Part model, mm, in its own coordinate system. Face numbers are marked on the shaded views. A direction names the side the tool comes from. Give positions to 0.01 mm unless a question says otherwise; leave off trailing zeros. Order: outer loops, then holes, each group sorted by start corner. A loop starts at its lowest first (then second) coordinate and runs counter-clockwise, first axis right, second up. Notation, with made-up numbers: (48.5, -4) - (75.5, -4) arc R36 cw to (75.5, 34) - close; hole circle Ø5 at (-17.5, 19.25). An arc over 180 degrees is marked (long way). Use one line per item in the form item = value. Start each with the question number.
1. Pull direction X, two halves, no side cores. Call the marked faces 3, 4, 5 and 6: +X half, -X half, draft (parallel to the pull), parting line (faces both ways), or undercut.
2. Band-saw the part on B-B, the plane z = 0. List the corners of the cut face in (x, y).
3. Drill centre lines: line 1 (X direction, y = 21.25, z = 19.05); line 2 (Z direction, x = -10.5, y = 0.25); line 3 (X direction, y = 20.8, z = -38.1). Where is each one in solid material? Low to high.
4. Pin check, flat tips, straight feed: P1, Ø2.5, axis at y = 2.5, z = 33, coming from the +X side; P2, Ø4, axis at y = 2.5, z = 31, coming from the -X side; P3, Ø8, axis at x = 4.5, z = 36, coming from the +Y side; P4, Ø12, axis at x = 18.5, y = 17, coming from the -Z side. Stop position of each tip, or through.
5. Band-saw the part on D-D, the plane z = 30.5. List the corners of the cut face in (x, y) (3 decimals).
6. Tool access for the marked faces 1 and 2: list every direction of +Z, -Z, +X, -X, +Y, -Y with a clear straight run to the whole face (end or side of a thin tool).
7. Band-saw the part on C-C, the plane y = 10.75. State how many separate pieces and enclosed holes the cut face has, plus the area to 3 significant figures.
8. Band-saw the part on A-A, the plane x = 14.5. List the corners of the cut face in (y, z), plus the area to 3 significant figures.
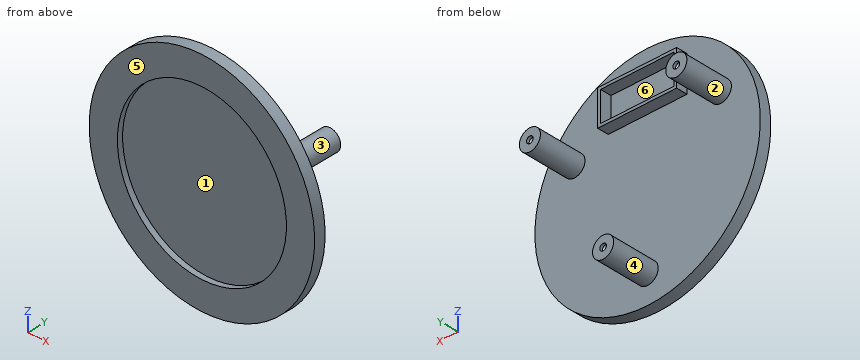
from build123d import *

# Parameters (mm, degrees)
SKETCH3_R                 = 4.7625
BOSS_EXTRUDE1_DEPTH       = 21.59
M4X0_7_TAPPED_HOLE1_D     = 3
M4X0_7_TAPPED_HOLE1_DEPTH = 1.27
M4X0_7_TAPPED_HOLE1_TIP   = 0.901290929
SKETCH12_W                = 35.54
SKETCH12_H                = 16.04
SKETCH12_W_2              = 33
SKETCH12_H_2              = 13.5
BOSS_EXTRUDE2_DEPTH       = 5.08


with BuildPart() as part:
    # Sketch1 → Revolve1 (revolve)
    with BuildSketch(Plane.XY, mode=Mode.PRIVATE) as revolve1_sk:
        Polygon((-38.1, -2.54), (0, -2.54), (0, 0), (-50.8, 0), (-50.8, -5.08), (-38.1, -5.08), align=None)
    revolve(revolve1_sk.sketch.rotate(Axis((0, 4.567685351, 0), (0, -1, 0)), 270), axis=Axis((0, 4.567685351, 0), (0, -1, 0)))

    # Sketch3 → Boss-Extrude1 (add)
    with BuildSketch(Plane(origin=(0, 0, 0), x_dir=(1, 0, 0), z_dir=(0, 1, 0))):
        with Locations(Location((0, 38.1, 0), (0, 0, 270))):
            Circle(SKETCH3_R)
        with Locations(Location((-32.995567884, -19.05, 0), (0, 0, 270))):
            Circle(SKETCH3_R)
        with Locations(Location((32.995567884, -19.05, 0), (0, 0, 270))):
            Circle(SKETCH3_R)
    extrude(amount=BOSS_EXTRUDE1_DEPTH)

    # M4x0.7 Tapped Hole1
    with Locations(Plane(origin=(0, 21.59, 0), x_dir=(1, 0, 0), z_dir=(0, 1, 0))):
        with Locations((-32.995567884, -19.05), (0, 38.1), (32.995567884, -19.05)):
            Hole(M4X0_7_TAPPED_HOLE1_D / 2, depth=M4X0_7_TAPPED_HOLE1_DEPTH)
            with Locations((0, 0, -(M4X0_7_TAPPED_HOLE1_DEPTH + M4X0_7_TAPPED_HOLE1_TIP / 2))):  # 118° drill point
                Cone(0, M4X0_7_TAPPED_HOLE1_D / 2, M4X0_7_TAPPED_HOLE1_TIP, mode=Mode.SUBTRACT)

    # Sketch12 → Boss-Extrude2 (add)
    with BuildSketch(Plane(origin=(0, 0, 0), x_dir=(1, 0, 0), z_dir=(0, 1, 0))):
        with Locations((0, -32.723460825)):
            Rectangle(SKETCH12_W, SKETCH12_H)
        with Locations((0, -32.723460825)):
            Rectangle(SKETCH12_W_2, SKETCH12_H_2, mode=Mode.SUBTRACT)
    extrude(amount=BOSS_EXTRUDE2_DEPTH)


solid = part.part
From the geometry:
q1.face_3 = undercut
q1.face_4 = parting line
q1.face_5 = draft
q1.face_6 = undercut
q2.outline = (-50.8, -5.08) - (-38.1, -5.08) - (-38.1, -2.54) - (38.1, -2.54) - (38.1, -5.08) - (50.8, -5.08) - (50.8, 0) - (-50.8, 0) - close
q3.line_1 = -37.76 to -34.5, -31.5 to -28.23, 28.23 to 31.5, 34.5 to 37.76
q3.line_2 = 24.7 to 25.97, 39.47 to 40.74
q3.line_3 = -4.76 to -1.5, 1.5 to 4.76
q4.P1 = 17.77
q4.P2 = -17.77
q4.P3 = 5.08
q4.P4 = through
q5.outline = (-40.625, -5.08) - (-22.833, -5.08) - (-22.833, -2.54) - (22.833, -2.54) - (22.833, -5.08) - (40.625, -5.08) - (40.625, 0) - (17.77, 0) - (17.77, 5.08) - (16.5, 5.08) - (16.5, 0) - (-16.5, 0) - (-16.5, 5.08) - (-17.77, 5.08) - (-17.77, 0) - (-40.625, 0) - close
q6.face_1 = -Y
q6.face_2 = +Y
q7.separate_pieces = 3
q7.enclosed_holes = 0
q7.area = 214 mm²
q8.outline = (-5.08, -48.69) - (0, -48.69) - (0, 24.7) - (5.08, 24.7) - (5.08, 25.97) - (0, 25.97) - (0, 39.47) - (5.08, 39.47) - (5.08, 40.74) - (0, 40.74) - (0, 48.69) - (-5.08, 48.69) - (-5.08, 35.23) - (-2.54, 35.23) - (-2.54, -35.23) - (-5.08, -35.23) - close
q8.area = 329 mm²
